The model under review builds one solid part; all positions refer to its coordinate system, in mm. A direction names the side the tool comes from. Give positions to 0.01 mm unless a question says otherwise; leave off trailing zeros. Write each loop counter-clockwise with the first axis right and the second up, starting at its lowest first coordinate (ties: lowest second). Pieces come first, ordered by that corner, then holes.
from build123d import *

# Parameters (mm, degrees)
BOSS_EXTRUDE1_DEPTH = 10
SKETCH2_R           = 3.75
CUT_EXTRUDE1_DEPTH  = 8
SKETCH3_R           = 3
CUT_EXTRUDE2_DEPTH  = 3


with BuildPart() as part:
    # Sketch1 → Boss-Extrude1 (new body, symmetric)
    with BuildSketch(Plane.XY):
        Polygon((-6, 10), (-6, 6.45), (-8, 6.45), (-8, 3.55), (-6, 3.55), (-6, 0), (6, 0), (6, 3.55), (8, 3.55), (8, 6.45), (6, 6.45), (6, 10), align=None)
    extrude(amount=BOSS_EXTRUDE1_DEPTH, both=True)

    # Sketch2 → Cut-Extrude1 (cut)
    with BuildSketch(Plane(origin=(0, 10, 0), x_dir=(1, 0, 0), z_dir=(0, 1, 0))):
        Circle(SKETCH2_R)
    extrude(amount=-CUT_EXTRUDE1_DEPTH, mode=Mode.SUBTRACT)

    # Sketch3 → Cut-Extrude2 (cut, through all)
    with BuildSketch(Plane(origin=(0, 2, 0), x_dir=(1, 0, 0), z_dir=(0, 1, 0))):
        Circle(SKETCH3_R)
    extrude(amount=-CUT_EXTRUDE2_DEPTH, mode=Mode.SUBTRACT)


solid = part.part
1) Insertion check: pin 1 (3 mm diameter, centred on y = 8.5, z = -5, fed in from -X); pin 2 (1.5 mm diameter, centred on x = 2, z = 6, fed in from -Y); pin 3 (3 mm diameter, centred on y = 1.5, z = 0, fed in from +X); pin 4 (1 mm diameter, centred on x = 7.5, z = -1.5, fed in from -Y). Each pin has a flat end and moves straight along its axis. Give the tip position at first contact, or say it passes through.
2) To check wall thickness, follow probe 1 along Z at (x, y) = (0, 5); probe 2 along X at (y, z) = (5.5, 0); probe 3 along X at (y, z) = (8, 0). State the ranges of each line that lie inside material, in increasing order.
3) Tool access review of faces 4 (the flat face through (-7, 3.55, 0)), 5 (the flat face through (7, 6.45, 0)), 6 (the cylindrical face through (-3.746, 6.056, -0.165)): name each direction out of +Z, -Z, +X, -X, +Y, -Y from which nothing blocks a thin tool from reaching the whole face with its end or side.
4) Consider section B-B, the plane z = 0. Give the boundary of the cut face in (x, y), then the cut area to 3 significant figures.
5) The part is to be moulded in two halves that separate along X. For faces 1 (the flat face through (6, 2, 0)), 2 (the flat face through (1, 2, -3)), 3 (the flat face through (7, 3.55, 0)), say which applies: +X half, -X half, draft (parallel to the pull), parting line (faces both ways), or undercut.
6) Consider section D-D, the plane z = -7.5. Give the boundary of the cut face in (x, y).
7) Consider section A-A, the plane x = 0. Give the boundary of the cut face in (y, z).
8) Consider section C-C, the plane y = 2.25. Give the boundary of the cut face in (x, z), then the cut area to 3 significant figures.
Answer block:
1. pin 1: stops at x = -6
1. pin 2: stops at y = 0
1. pin 3: stops at x = 6
1. pin 4: stops at y = 3.55
2. probe 1: z = -10 to -3.75, 3.75 to 10
2. probe 2: x = -8 to -3.75, 3.75 to 8
2. probe 3: x = -6 to -3.75, 3.75 to 6
3. face 4: +Z, -Z, -X, -Y
3. face 5: +Z, -Z, +X, +Y
3. face 6: +Y
4. outline: (-8, 3.55) - (-6, 3.55) - (-6, 0) - (-3, 0) - (-3, 2) - (-3.75, 2) - (-3.75, 10) - (-6, 10) - (-6, 6.45) - (-8, 6.45) - close; (3, 0) - (6, 0) - (6, 3.55) - (8, 3.55) - (8, 6.45) - (6, 6.45) - (6, 10) - (3.75, 10) - (3.75, 2) - (3, 2) - close
4. area: 59.6 mm2
5. face 1: +X half
5. face 2: undercut
5. face 3: draft
6. outline: (-8, 3.55) - (-6, 3.55) - (-6, 0) - (6, 0) - (6, 3.55) - (8, 3.55) - (8, 6.45) - (6, 6.45) - (6, 10) - (-6, 10) - (-6, 6.45) - (-8, 6.45) - close
7. outline: (0, -10) - (10, -10) - (10, -3.75) - (2, -3.75) - (2, -3) - (0, -3) - close; (0, 3) - (2, 3) - (2, 3.75) - (10, 3.75) - (10, 10) - (0, 10) - close
8. outline: (-6, -10) - (6, -10) - (6, 10) - (-6, 10) - close; hole circle Ø7.5 at (0, 0)
8. area: 196 mm2
